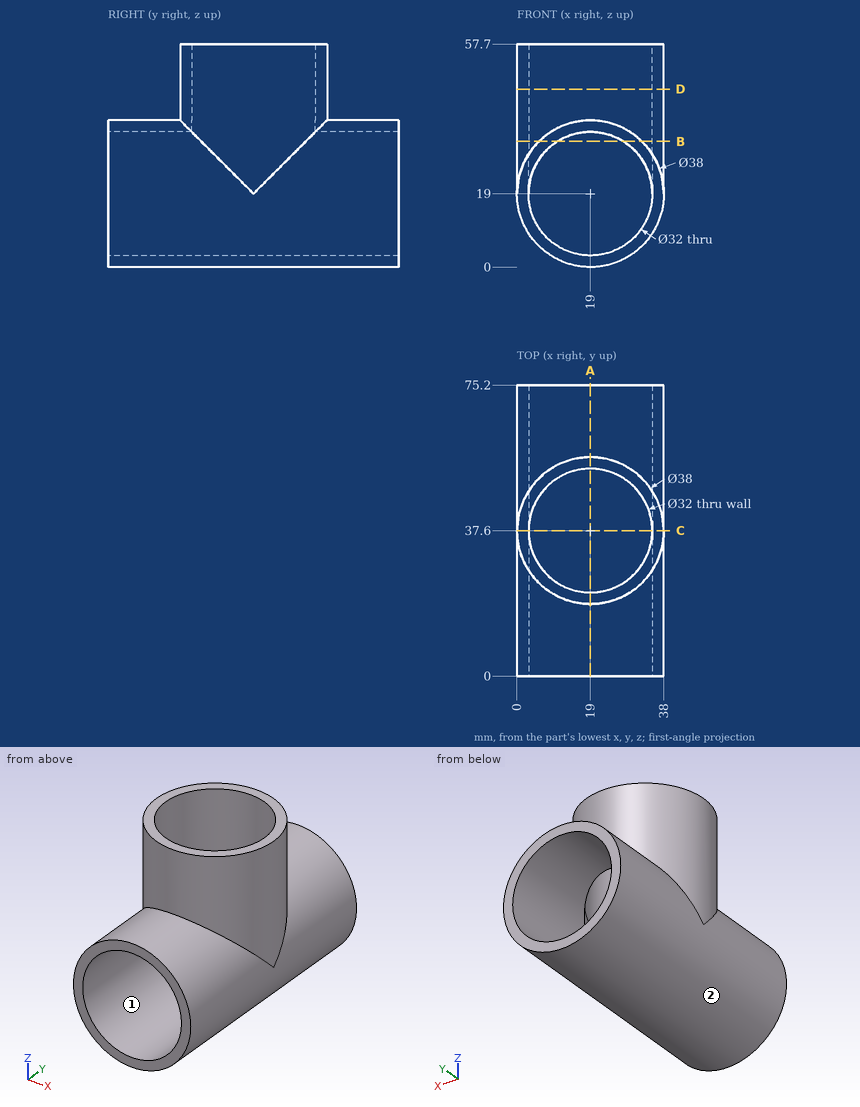
For this review, use the dimensioned drawing (mm, ordinates from the lowest corner) and the shaded views. Round coordinates to 2 decimals unless told otherwise and drop trailing zeros. Order: outer loops, then holes, each group sorted by start corner. A loop starts at its lowest first (then second) coordinate and runs counter-clockwise, first axis right, second up. Notation, with made-up numbers: M 65.5,86.5 L 115.5,86.5 A26 ccw 115.5,118.5 Z; hole C -14.5,45 d3. An arc over 180 degrees is marked long. Use a Markdown table: item, result. Add a question column.
Item 1: Add section B-B, the plane z = 32.5. Give the boundary of the cut face in (x, y).
Item 2: Insertion check: pin 1 (5 mm diameter, centred on x = 28.5, y = 16.5, fed in from +Z); pin 2 (1.5 mm diameter, centred on x = 8, z = 50.5, fed in from +Y); pin 3 (1.5 mm diameter, centred on y = 48, z = 16.5, fed in from -X). Each pin has a flat end and moves straight along its axis. Give the tip position at first contact, or say it passes through.
Item 3: Add section D-D, the plane z = 46. Give the boundary of the cut face in (x, y).
Item 4: Mouldability with a two-part tool opening along X and no side actions: class the marked faces 1 and 2 as released by +X, released by -X, zero draft, split by the parting line, or undercut.
Item 5: To check wall thickness, follow line 1 along X through (y, z) = (39.5, 19); line 2 along Y through (x, z) = (19, 41.25); line 3 along Z through (x, y) = (27.5, 60.5). State the ranges of each line that lie inside material, in increasing order.
Item 6: Add section C-C, the plane y = 37.6. Give the boundary of the cut face in (x, z).
Item 7: Add section A-A, the plane x = 19. Give the boundary of the cut face in (y, z).
Geometry results:
| question | item | result |
|---|---|---|
| 1 | outline | M 5.63,0 L 10.41,0 L 10.41,24.1 A16 cw 10.41,51.1 L 10.41,75.2 L 5.63,75.2 L 5.63,51.1 A19 ccw 5.63,24.1 Z; M 27.59,0 L 32.37,0 L 32.37,24.1 A19 ccw 32.37,51.1 L 32.37,75.2 L 27.59,75.2 L 27.59,51.1 A16 cw 27.59,24.1 Z |
| 2 | pin 1 | stops at z = 36.66 |
| 2 | pin 2 | stops at y = 53.6 |
| 2 | pin 3 | stops at x = 0.08 |
| 3 | outline | C 19,37.6 d38; hole C 19,37.6 d32 |
| 4 | face 1 | undercut |
| 4 | face 2 | split by the parting line |
| 5 | line 1 | x = 0 to 3, 35 to 38 |
| 5 | line 2 | y = 18.6 to 21.6, 53.6 to 56.6 |
| 5 | line 3 | z = 2.01 to 5.44, 32.56 to 35.99 |
| 6 | outline | M 0,19 A19 ccw 38,19 L 38,57.7 L 35,57.7 L 35,19 A16 cw 3,19 L 3,57.7 L 0,57.7 Z |
| 7 | outline | M 0,0 L 75.2,0 L 75.2,3 L 0,3 Z; M 0,35 L 21.6,35 L 21.6,57.7 L 18.6,57.7 L 18.6,38 L 0,38 Z; M 53.6,35 L 75.2,35 L 75.2,38 L 56.6,38 L 56.6,57.7 L 53.6,57.7 Z |
